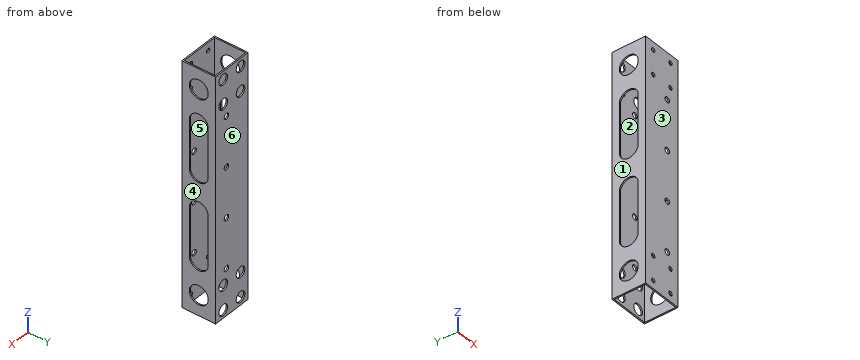
from build123d import *

# Parameters (mm, degrees)
SKETCH_1_W          = 30
SKETCH_1_H          = 25
SKETCH_1_W_2        = 28
SKETCH_1_H_2        = 23
EXTRUDE_1_DEPTH     = 90
SKETCH_2_R          = 2.1
CUT_EXTRUDE_1_DEPTH = 30
SKETCH_3_R          = 1.55
CUT_EXTRUDE_2_DEPTH = 30
SKETCH_4_R          = 4
CUT_EXTRUDE_3_DEPTH = 10
SKETCH_5_R          = 7
CUT_EXTRUDE_4_DEPTH = 30


with BuildPart() as part:
    # 草图1 → 凸台-拉伸1 (new, symmetric)
    with BuildSketch(Plane.XY):
        Rectangle(SKETCH_1_W, SKETCH_1_H)
        Rectangle(SKETCH_1_W_2, SKETCH_1_H_2, mode=Mode.SUBTRACT)
    extrude(amount=EXTRUDE_1_DEPTH, both=True)

    # 草图2 → 切除-拉伸1 (cut)
    with BuildSketch(Plane(origin=(0, 12.5, 0), x_dir=(1, 0, 0), z_dir=(0, 1, 0))):
        with Locations(Location((5, 55.51, 0), (0, 0, 180))):
            Circle(SKETCH_2_R)
        with Locations(Location((5, -55.49, 0), (0, 0, 180))):
            Circle(SKETCH_2_R)
        with Locations(Location((5, -18.49, 0), (0, 0, 180))):
            Circle(SKETCH_2_R)
        with Locations(Location((5, 18.51, 0), (0, 0, 180))):
            Circle(SKETCH_2_R)
    extrude(amount=-CUT_EXTRUDE_1_DEPTH, mode=Mode.SUBTRACT)

    # 草图3 → 切除-拉伸2 (cut)
    with BuildSketch(Plane(origin=(0, 12.5, 0), x_dir=(1, 0, 0), z_dir=(0, 1, 0))):
        with Locations(Location((8, 84, 0), (0, 0, 180))):
            Circle(SKETCH_3_R)
        with Locations(Location((8, 66, 0), (0, 0, 180))):
            Circle(SKETCH_3_R)
        with Locations(Location((-8, 84, 0), (0, 0, 180))):
            Circle(SKETCH_3_R)
        with Locations(Location((-8, 66, 0), (0, 0, 180))):
            Circle(SKETCH_3_R)
        with Locations(Location((8, -66, 0), (0, 0, 180))):
            Circle(SKETCH_3_R)
        with Locations(Location((-8, -66, 0), (0, 0, 180))):
            Circle(SKETCH_3_R)
        with Locations(Location((-8, -84, 0), (0, 0, 180))):
            Circle(SKETCH_3_R)
        with Locations(Location((8, -84, 0), (0, 0, 180))):
            Circle(SKETCH_3_R)
    extrude(amount=-CUT_EXTRUDE_2_DEPTH, mode=Mode.SUBTRACT)

    # 草图4 → 切除-拉伸3 (cut)
    with BuildSketch(Plane(origin=(0, 12.5, 0), x_dir=(1, 0, 0), z_dir=(0, 1, 0))):
        with Locations(Location((8, -84, 0), (0, 0, 180))):
            Circle(SKETCH_4_R)
        with Locations(Location((-8, -84, 0), (0, 0, 180))):
            Circle(SKETCH_4_R)
        with Locations(Location((-8, -66, 0), (0, 0, 180))):
            Circle(SKETCH_4_R)
        with Locations(Location((8, -66, 0), (0, 0, 180))):
            Circle(SKETCH_4_R)
        with Locations(Location((-8, 66, 0), (0, 0, 180))):
            Circle(SKETCH_4_R)
        with Locations(Location((8, 66, 0), (0, 0, 180))):
            Circle(SKETCH_4_R)
        with Locations(Location((8, 84, 0), (0, 0, 180))):
            Circle(SKETCH_4_R)
        with Locations(Location((-8, 84, 0), (0, 0, 180))):
            Circle(SKETCH_4_R)
    extrude(amount=-CUT_EXTRUDE_3_DEPTH, mode=Mode.SUBTRACT)

    # 草图5 → 切除-拉伸4 (cut)
    with BuildSketch(Plane.ZY.offset(15)):
        with Locations(Location((75, 0, 0), (0, 0, 270))):
            Circle(SKETCH_5_R)
        with Locations(Location((-75, 0, 0), (0, 0, 180))):
            Circle(SKETCH_5_R)
        with BuildLine():
            Line((14, 7), (50, 7))
            ThreePointArc((50, 7), (57, 0), (50, -7))
            Line((50, -7), (14, -7))
            ThreePointArc((14, -7), (7, 0), (14, 7))
        make_face()
        with BuildLine():
            Line((-14, 7), (-50, 7))
            ThreePointArc((-50, 7), (-57, 0), (-50, -7))
            Line((-50, -7), (-14, -7))
            ThreePointArc((-14, -7), (-7, 0), (-14, 7))
        make_face()
    extrude(amount=-CUT_EXTRUDE_4_DEPTH, mode=Mode.SUBTRACT)


solid = part.part
Input: part model. Units: mm. Frame: model coordinates. Face numbers are marked on the shaded views. A direction names the side the tool comes from. Coordinates: 2 decimals unless noted, no trailing zeros. Loops run counter-clockwise (first coordinate to the right, second up) from the corner with the lowest first, then second, coordinate; pieces in that order, holes last. Notation, with made-up numbers: (-7.5, -23) -> (25.5, -23) arc R10 cw to (25.5, -13) -> close; hole circle Ø10 at (-1, 26). An arc over 180 degrees is marked (long way). Write item = value, one per line. Start each with the question number.
Item 1: Cut plane D-D, the plane z = -18.51. Return loops of the section in (x, y).
Item 2: Cut plane C-C, the plane y = 8.5. Return loops of the section in (x, z).
Item 3: Mould query, pull axis X, two halves, no side actions, for the marked faces 1, 2, 3 and 4. Classes: pulls with the +X half, pulls with the -X half, needs draft (parallel to the pull), parting line crosses it, or undercut.
Item 4: Material intervals for line 1 (X direction, y = -11.9, z = -84); line 2 (Z direction, x = -8, y = -12.3); line 3 (X direction, y = 10, z = 23.5), sorted ascending.
Item 5: Cut plane A-A, the plane z = -84. Return loops of the section in (x, y).
Item 6: First-contact query: P1, Ø6.5, axis at x = 8, z = 84, coming from the +Y side. Flat tip, straight axial feed; report the tip coordinate or a pass-through.
Item 7: Reachability of the marked faces 5 and 6 from +Z, -Z, +X, -X, +Y, -Y: full face, straight path, thin tool, end or side. Return the list, or none.
Item 8: Cut plane B-B, the plane z = 41. Return loops of the section in (x, y), plus the area to 3 significant figures.
Ans:
q1.outline = (-15, -12.5) -> (2.9, -12.5) -> (2.9, -11.5) -> (-14, -11.5) -> (-14, -7) -> (-15, -7) -> close; (-15, 7) -> (-14, 7) -> (-14, 11.5) -> (2.9, 11.5) -> (2.9, 12.5) -> (-15, 12.5) -> close; (7.1, -12.5) -> (15, -12.5) -> (15, -7) -> (14, -7) -> (14, -11.5) -> (7.1, -11.5) -> close; (7.1, 11.5) -> (14, 11.5) -> (14, 7) -> (15, 7) -> (15, 12.5) -> (7.1, 12.5) -> close
q2.outline = (-15, -90) -> (-14, -90) -> (-14, 90) -> (-15, 90) -> close; (14, -90) -> (15, -90) -> (15, 90) -> (14, 90) -> close
q3.face_1 = pulls with the -X half
q3.face_2 = undercut
q3.face_3 = needs draft
q3.face_4 = pulls with the +X half
q4.line_1 = -15 to -9.55, -6.45 to 6.45, 9.55 to 15
q4.line_2 = -90 to -85.55, -82.45 to -67.55, -64.45 to 64.45, 67.55 to 82.45, 85.55 to 90
q4.line_3 = -15 to -14, 14 to 15
q5.outline = (-15, -12.5) -> (-9.55, -12.5) -> (-9.55, -11.5) -> (-14, -11.5) -> (-14, 11.5) -> (-12, 11.5) -> (-12, 12.5) -> (-15, 12.5) -> close; (-6.45, -12.5) -> (6.45, -12.5) -> (6.45, -11.5) -> (-6.45, -11.5) -> close; (-4, 11.5) -> (4, 11.5) -> (4, 12.5) -> (-4, 12.5) -> close; (9.55, -12.5) -> (15, -12.5) -> (15, 12.5) -> (12, 12.5) -> (12, 11.5) -> (14, 11.5) -> (14, -11.5) -> (9.55, -11.5) -> close
q6.P1 = -11.5
q7.face_5 = +Z, -Z
q7.face_6 = +Z, -Z, +X, -X, +Y
q8.outline = (-15, -12.5) -> (15, -12.5) -> (15, -7) -> (14, -7) -> (14, -11.5) -> (-14, -11.5) -> (-14, -7) -> (-15, -7) -> close; (-15, 7) -> (-14, 7) -> (-14, 11.5) -> (14, 11.5) -> (14, 7) -> (15, 7) -> (15, 12.5) -> (-15, 12.5) -> close
q8.area = 78.0 mm²
